```python
from build123d import *

# Parameters (mm, degrees)
RESSALTO_EXTRUS_O2_DEPTH = 6.75
ESBO_O3_W                = 20.7
ESBO_O3_H                = 8.969000478
CORTE_EXTRUS_O1_DEPTH    = 2.75
ESBO_O4_W                = 20.7
ESBO_O4_H                = 8.969000478
CORTE_EXTRUS_O2_DEPTH    = 2.75
ESBO_O5_W                = 34
ESBO_O5_H                = 19.5
CORTE_EXTRUS_O3_DEPTH    = 1.55
ESBO_O6_W                = 34
ESBO_O6_H                = 19.5
CORTE_EXTRUS_O4_DEPTH    = 1.55
ESBO_O8_W                = 3.076935564
ESBO_O8_H                = 19
ESBO_O8_W_2              = 3.076935565
CORTE_EXTRUS_O5_DEPTH    = 1.7
ESBO_O9_W                = 3.076935565
ESBO_O9_H                = 19
ESBO_O9_W_2              = 3.076935564
CORTE_EXTRUS_O6_DEPTH    = 1.7
ESBO_O10_W               = 9
ESBO_O10_H               = 21.7
ESBO_O10_W_2             = 8
ESBO_O10_H_2             = 20.7
CORTE_EXTRUS_O7_DEPTH    = 1
ESBO_O11_W               = 6.4
ESBO_O11_H               = 0.8
RESSALTO_EXTRUS_O3_DEPTH = 10.3
ESBO_O12_R               = 1.5
CORTE_EXTRUS_O8_DEPTH    = 43.061413316
CHANFRO1_SIZE            = 1


with BuildPart() as part:
    # Esboço1 → Ressalto-extrusão2 (new, symmetric)
    with BuildSketch(Plane(origin=(0, 0, 0), x_dir=(0, 0, -1), z_dir=(1, 0, 0))):
        with BuildLine():
            Line((0, 0), (27.846128871, 0))
            Line((27.846128871, 0), (30.923064436, 13.5))
            Line((30.923064436, 13.5), (30.923064436, 19))
            Line((30.923064436, 19), (29.923064436, 19))
            Line((29.923064436, 19), (29.923064436, 13.612517806))
            Line((29.923064436, 13.612517806), (27.846128871, 4.5))
            Line((27.846128871, 4.5), (27.846128871, 19.5))
            Line((27.846128871, 19.5), (29.273064436, 19.5))
            Line((29.273064436, 19.5), (29.273064436, 21.5))
            Line((29.273064436, 21.5), (24.273064436, 21.5))
            ThreePointArc((24.273064436, 21.5), (16.071387559, 23.940840139), (10.5389083, 30.469000478))
            ThreePointArc((10.5389083, 30.469000478), (5.927855619, 26.860671745), (3.573064436, 21.5))
            Line((3.573064436, 21.5), (-1.426935564, 21.5))
            Line((-1.426935564, 21.5), (-1.426935564, 19.5))
            Line((-1.426935564, 19.5), (0, 19.5))
            Line((0, 19.5), (0, 4.5))
            Line((0, 4.5), (-2.076935564, 13.612517806))
            Line((-2.076935564, 13.612517806), (-2.076935564, 19))
            Line((-2.076935564, 19), (-3.076935564, 19))
            Line((-3.076935564, 19), (-3.076935564, 13.5))
            Line((-3.076935564, 13.5), (0, 0))
        make_face()
    extrude(amount=RESSALTO_EXTRUS_O2_DEPTH, both=True)

    # Esboço3 → Corte-extrusão1 (cut)
    with BuildSketch(Plane(origin=(6.75, 0, 0), x_dir=(0, 0, -1), z_dir=(1, 0, 0))):
        with Locations((13.923064436, 25.984500239)):
            Rectangle(ESBO_O3_W, ESBO_O3_H)
    extrude(amount=-CORTE_EXTRUS_O1_DEPTH, mode=Mode.SUBTRACT)

    # Esboço4 → Corte-extrusão2 (cut)
    with BuildSketch(Plane.ZY.offset(6.75)):
        with Locations((-13.923064436, 25.984500239)):
            Rectangle(ESBO_O4_W, ESBO_O4_H)
    extrude(amount=-CORTE_EXTRUS_O2_DEPTH, mode=Mode.SUBTRACT)

    # Esboço5 → Corte-extrusão3 (cut)
    with BuildSketch(Plane.ZY.offset(6.75)):
        with Locations((-13.923064436, 9.75)):
            Rectangle(ESBO_O5_W, ESBO_O5_H)
    extrude(amount=-CORTE_EXTRUS_O3_DEPTH, mode=Mode.SUBTRACT)

    # Esboço6 → Corte-extrusão4 (cut)
    with BuildSketch(Plane(origin=(6.75, 0, 0), x_dir=(0, 0, -1), z_dir=(1, 0, 0))):
        with Locations((13.923064436, 9.75)):
            Rectangle(ESBO_O6_W, ESBO_O6_H)
    extrude(amount=-CORTE_EXTRUS_O4_DEPTH, mode=Mode.SUBTRACT)

    # Esboço8 → Corte-extrusão5 (cut)
    with BuildSketch(Plane(origin=(5.2, 0, 0), x_dir=(0, 0, -1), z_dir=(1, 0, 0))):
        with Locations((-1.538467782, 9.5)):
            Rectangle(ESBO_O8_W, ESBO_O8_H)
        with Locations((29.384596654, 9.5)):
            Rectangle(ESBO_O8_W_2, ESBO_O8_H)
    extrude(amount=-CORTE_EXTRUS_O5_DEPTH, mode=Mode.SUBTRACT)

    # Esboço9 → Corte-extrusão6 (cut)
    with BuildSketch(Plane.ZY.offset(5.2)):
        with Locations((-29.384596654, 9.5)):
            Rectangle(ESBO_O9_W, ESBO_O9_H)
        with Locations((1.538467782, 9.5)):
            Rectangle(ESBO_O9_W_2, ESBO_O9_H)
    extrude(amount=-CORTE_EXTRUS_O6_DEPTH, mode=Mode.SUBTRACT)

    # Esboço10 → Corte-extrusão7 (cut)
    with BuildSketch(Plane(origin=(0, 21.5, 0), x_dir=(1, 0, 0), z_dir=(0, 1, 0))):
        with Locations((0, 13.923064436)):
            Rectangle(ESBO_O10_W, ESBO_O10_H)
        with Locations((0, 13.923064436)):
            Rectangle(ESBO_O10_W_2, ESBO_O10_H_2, mode=Mode.SUBTRACT)
    extrude(amount=-CORTE_EXTRUS_O7_DEPTH, mode=Mode.SUBTRACT)

    # Esboço11 → Ressalto-extrusão3 (add)
    with BuildSketch(Plane.XZ):
        with Locations((0, -3.123064436)):
            Rectangle(ESBO_O11_W, ESBO_O11_H)
        with Locations((0, -13.923064436)):
            Rectangle(ESBO_O11_W, ESBO_O11_H)
        with Locations((0, -24.723064436)):
            Rectangle(ESBO_O11_W, ESBO_O11_H)
    extrude(amount=RESSALTO_EXTRUS_O3_DEPTH)

    # Esboço12 → Corte-extrusão8 (cut, through all)
    with BuildSketch(Plane(origin=(0, 0, -25.123064436), x_dir=(-1, 0, 0), z_dir=(0, 0, -1))):
        with Locations((0, -5.3)):
            Circle(ESBO_O12_R)
    extrude(amount=-CORTE_EXTRUS_O8_DEPTH, mode=Mode.SUBTRACT)

    # Chanfro1
    chanfro1_edges = [part.edges().sort_by_distance(p)[0] for p in [
        (-3.2, -10.3, -3.123064436),
        (3.2, -10.3, -3.123064436),
        (-3.2, -10.3, -13.923064436),
        (3.2, -10.3, -13.923064436),
        (-3.2, -10.3, -24.723064436),
        (3.2, -10.3, -24.723064436),
    ]]
    chamfer(chanfro1_edges, length=CHANFRO1_SIZE)


solid = part.part
```
Check sheet for the modelled part. Datum: model origin and axes. Units: mm. A direction names the side the tool comes from. Round coordinates to 2 decimals unless told otherwise and drop trailing zeros. Order: outer loops, then holes, each group sorted by start corner. A loop starts at its lowest first (then second) coordinate and runs counter-clockwise, first axis right, second up. Notation, with made-up numbers: (42, 78.25) -> (74, 78.25) arc R28 cw to (74, 109.25) -> close; hole circle Ø11 at (50, -25). An arc over 180 degrees is marked (long way). One line per item, written item: value. Start each with the question number.
Q1. Set-up check for faces 4 (the face through (-4, 23, -11)), 5 (the face through (0, 16, 2.077)), 6 (the face through (-2.7, -9.8, -3.1)): record each of +Z, -Z, +X, -X, +Y, -Y from which the full face is reachable in a straight line by a thin tool's end or side.
Q2. Gauge pin test, flat ends, axial feed: pin 1 Ø1 at (x, y) = (-2, 20.5) entering from +Z; pin 2 Ø0.6 at (x, y) = (-1, 20) entering from -Z; pin 3 Ø3.5 at (x, y) = (0, -5.3) entering from -Z. Record the tip position at first contact, or that the pin passes through.
Q3. Thickness scan on line 1 (Z direction, x = 2.25, y = 18); line 2 (Z direction, x = 1, y = -1); line 3 (Y direction, x = 0, z = -3.2). Record the ranges inside material, lowest first.
Q4. Cross-section at D-D (z = -5.5). Record the boundary of the cut face in (x, y), and give its area (3 significant figures).
Q5. Cross-section at C-C (x = 0). Give the number of separate pieces and of enclosed holes in the cut face, and give its area (3 significant figures).
Q6. Cross-section at A-A (y = 16.5). Record the boundary of the cut face in (x, z), and give its area (3 significant figures).
Q7. Cross-section at B-B (y = -5.3). Record the boundary of the cut face in (x, z), and give its area (3 significant figures).
Q8. Mould release check, pull along Y, two halves, no side actions. Record for faces 1 (the face through (0, 16, 3.077)), 2 (the face through (0, 12, 0)), 3 (the face through (2.7, -9.8, -13.9)): pulls with the +Y half, pulls with the -Y half, needs draft (parallel to the pull), parting line crosses it, or undercut.
Completed:
1. face 4: +Y
1. face 5: +X, -X, +Y
1. face 6: +Z, -Z, -X, -Y
2. pin 1: stops at z = 1.43
2. pin 2: stops at z = -29.27
2. pin 3: stops at z = -25.12
3. line 1: z = -30.92 to -29.92, -27.85 to 0, 2.08 to 3.08
3. line 2: z = -25.12 to -24.32, -14.32 to -13.52, -3.52 to -2.72
3. line 3: y = -10.3 to -6.8, -3.8 to 20.5
4. outline: (-6.75, 19.5) -> (-5.2, 19.5) -> (-5.2, 0) -> (5.2, 0) -> (5.2, 19.5) -> (6.75, 19.5) -> (6.75, 21.5) -> (4.5, 21.5) -> (4.5, 20.5) -> (4, 20.5) -> (4, 26.27) -> (-4, 26.27) -> (-4, 20.5) -> (-4.5, 20.5) -> (-4.5, 21.5) -> (-6.75, 21.5) -> close
4. area: 267 mm²
5. separate pieces: 4
5. enclosed holes: 0
5. area: 732 mm²
6. outline: (-5.2, -27.85) -> (5.2, -27.85) -> (5.2, 0) -> (-5.2, 0) -> close; (-3.5, -30.92) -> (3.5, -30.92) -> (3.5, -29.92) -> (-3.5, -29.92) -> close; (-3.5, 2.08) -> (3.5, 2.08) -> (3.5, 3.08) -> (-3.5, 3.08) -> close
6. area: 304 mm²
7. outline: (-3.2, -25.12) -> (-1.5, -25.12) -> (-1.5, -24.32) -> (-3.2, -24.32) -> close; (-3.2, -14.32) -> (-1.5, -14.32) -> (-1.5, -13.52) -> (-3.2, -13.52) -> close; (-3.2, -3.52) -> (-1.5, -3.52) -> (-1.5, -2.72) -> (-3.2, -2.72) -> close; (1.5, -25.12) -> (3.2, -25.12) -> (3.2, -24.32) -> (1.5, -24.32) -> close; (1.5, -14.32) -> (3.2, -14.32) -> (3.2, -13.52) -> (1.5, -13.52) -> close; (1.5, -3.52) -> (3.2, -3.52) -> (3.2, -2.72) -> (1.5, -2.72) -> close
7. area: 8.16 mm²
8. face 1: needs draft
8. face 2: undercut
8. face 3: pulls with the -Y half
